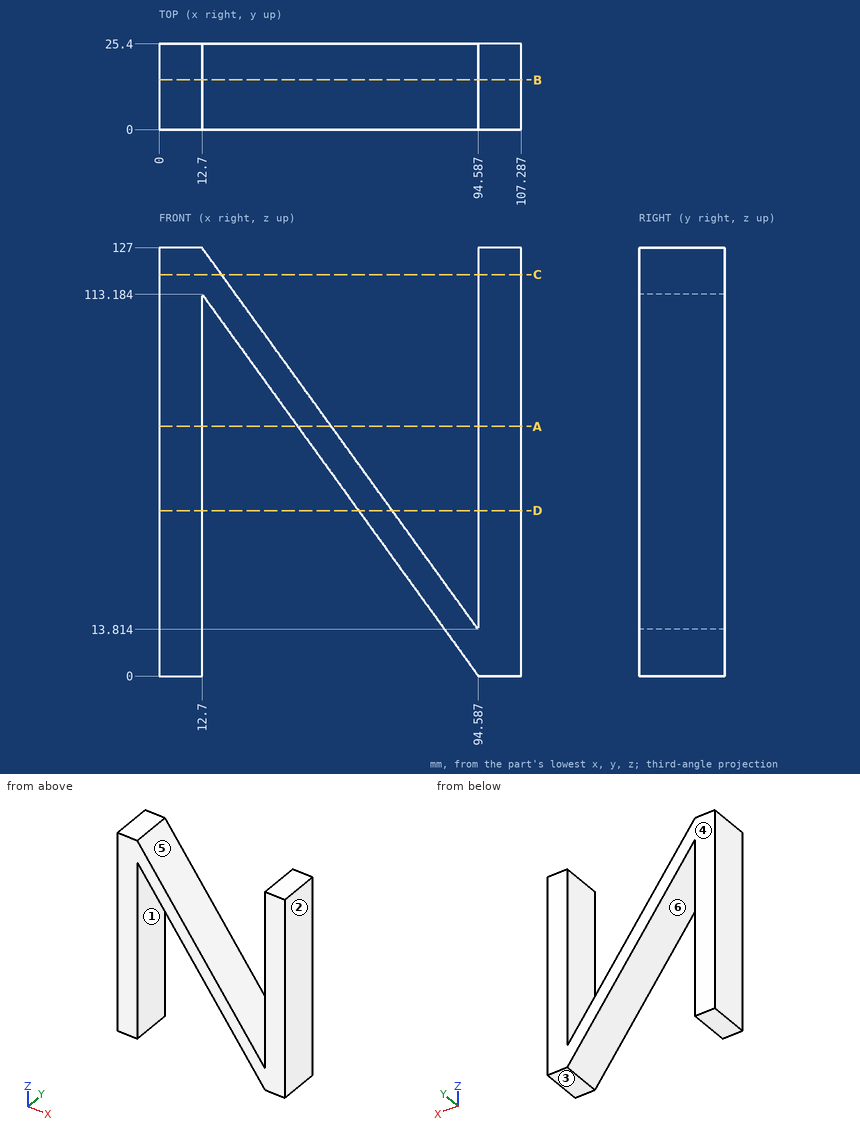
Could you check a few things on this drawing? It's one solid part, dimensions in mm from its lowest x, y, z. A direction names the side the tool comes from. Give positions to 0.01 mm unless a question says otherwise; leave off trailing zeros. Order: outer loops, then holes, each group sorted by start corner. A loop starts at its lowest first (then second) coordinate and runs counter-clockwise, first axis right, second up. Notation, with made-up numbers: (50.5, 1) - (83.5, 1) arc R20 cw to (83.5, 22) - close; hole circle Ø2 at (41, 79). An arc over 180 degrees is marked (long way). One line per question, with ' | ' between items. Start each with the question number.
Item 1: I want a section at B-B on y = 14.75. Write out the boundary of the cut face in (x, z), then the cut area to 3 significant figures.
Item 2: For the marked faces 4, 5 and 6, which set-ups out of +Z, -Z, +X, -X, +Y, -Y let a thin tool reach every point of the face, with its end or its side?
Item 3: I want a section at D-D on z = 49. Write out the boundary of the cut face in (x, y).
Item 4: I want a section at C-C on z = 119. Write out the boundary of the cut face in (x, y), then the cut area to 3 significant figures.
Item 5: I'm going to push flat-ended pins straight in: pin 1 Ø5 at (x, y) = (47, 9.5) entering from -Z; pin 2 Ø5 at (x, z) = (91.5, 73) entering from +Y. Where does each tip first touch, or does it pass through?
Item 6: I want a section at A-A on z = 74. Write out the boundary of the cut face in (x, y), then the cut area to 3 significant figures.
Item 7: Thinking about a two-plate mould opening in X: for the marked faces 1, 2 and 3, which applies, pulls with the +X half, pulls with the -X half, needs draft (parallel to the pull), parting line crosses it, or undercut?
Item 8: I need wall thicknesses on probe 1 along X at (y, z) = (7.75, 88) (1 decimal); probe 2 along X at (y, z) = (9.25, 83.5) (1 decimal); probe 3 along X at (y, z) = (20.5, 120.5). Which ranges of each line are inside material? Lowest first, please. Write a range as [from, to].
Verdict:
1) outline: (0, 0) - (12.7, 0) - (12.7, 113.18) - (94.59, 0) - (107.29, 0) - (107.29, 127) - (94.59, 127) - (94.59, 13.81) - (12.7, 127) - (0, 127) - close | area: 4,360 mm^2
2) face 4: +Z, -Z, +X, -X, +Y | face 5: +Z, +Y, -Y | face 6: -Z, +Y, -Y
3) outline: (0, 0) - (12.7, 0) - (12.7, 25.4) - (0, 25.4) - close; (59.14, 0) - (69.13, 0) - (69.13, 25.4) - (59.14, 25.4) - close; (94.59, 0) - (107.29, 0) - (107.29, 25.4) - (94.59, 25.4) - close
4) outline: (0, 0) - (18.49, 0) - (18.49, 25.4) - (0, 25.4) - close; (94.59, 0) - (107.29, 0) - (107.29, 25.4) - (94.59, 25.4) - close | area: 792 mm^2
5) pin 1: z = 62.32 | pin 2: through
6) outline: (0, 0) - (12.7, 0) - (12.7, 25.4) - (0, 25.4) - close; (41.05, 0) - (51.04, 0) - (51.04, 25.4) - (41.05, 25.4) - close; (94.59, 0) - (107.29, 0) - (107.29, 25.4) - (94.59, 25.4) - close | area: 899 mm^2
7) face 1: undercut | face 2: pulls with the +X half | face 3: needs draft
8) probe 1: [0, 12.7], [30.9, 40.9], [94.6, 107.3] | probe 2: [0, 12.7], [34.2, 44.2], [94.6, 107.3] | probe 3: [0, 17.4], [94.59, 107.29]
